```python
from build123d import *

# Parameters (mm, degrees)
SKETCH2_W           = 325
SKETCH2_H           = 220
SKETCH2_R           = 7
SKETCH2_R_2         = 3
BOSS_EXTRUDE3_DEPTH = 15
SKETCH11_W          = 70
SKETCH11_H          = 90
SKETCH11_W_2        = 50
SKETCH11_H_2        = 75
CUT_EXTRUDE2_DEPTH  = 8
FILLET1_R           = 3
SKETCH4_R           = 5
CUT_EXTRUDE3_DEPTH  = 5
SKETCH12_R          = 3
CUT_EXTRUDE4_DEPTH  = 5


with BuildPart() as part:
    # Sketch2 → Boss-Extrude3 (new body)
    with BuildSketch(Plane(origin=(0, 0, 0), x_dir=(1, 0, 0), z_dir=(0, 1, 0))):
        with Locations((7.596919738, 0)):
            Rectangle(SKETCH2_W, SKETCH2_H)
        with Locations(Location((155.096919738, -95, 0), (0, 0, 270))):
            Circle(SKETCH2_R, mode=Mode.SUBTRACT)
        with Locations(Location((155.096919738, 95, 0), (0, 0, 270))):
            Circle(SKETCH2_R, mode=Mode.SUBTRACT)
        with Locations(Location((-104.903080262, -95, 0), (0, 0, 270))):
            Circle(SKETCH2_R, mode=Mode.SUBTRACT)
        with Locations(Location((-104.903080262, 95, 0), (0, 0, 90))):
            Circle(SKETCH2_R, mode=Mode.SUBTRACT)
        with Locations(Location((-24.903080262, 105, 0), (0, 0, 270))):
            Circle(SKETCH2_R_2, mode=Mode.SUBTRACT)
        with Locations(Location((75.096919738, 105, 0), (0, 0, 270))):
            Circle(SKETCH2_R_2, mode=Mode.SUBTRACT)
        with Locations(Location((75.096919738, -105, 0), (0, 0, 90))):
            Circle(SKETCH2_R_2, mode=Mode.SUBTRACT)
        with Locations(Location((-24.903080262, -105, 0), (0, 0, 90))):
            Circle(SKETCH2_R_2, mode=Mode.SUBTRACT)
        with Locations(Location((165.096919738, 35, 0), (0, 0, 270))):
            Circle(SKETCH2_R_2, mode=Mode.SUBTRACT)
        with Locations(Location((165.096919738, -35, 0), (0, 0, 90))):
            Circle(SKETCH2_R_2, mode=Mode.SUBTRACT)
    extrude(amount=-BOSS_EXTRUDE3_DEPTH)

    # Sketch11 → Cut-Extrude2 (cut)
    with BuildSketch(Plane.XZ.offset(15)):
        with Locations((-39.903080262, 50)):
            Rectangle(SKETCH11_W, SKETCH11_H)
        with Locations((40.096919738, 50)):
            Rectangle(SKETCH11_W, SKETCH11_H)
        Polygon((85.096919738, 95), (135.096919738, 95), (135.096919738, 80), (155.096919738, 80), (155.096919738, 5), (85.096919738, 5), align=None)
        Polygon((85.096919738, -95), (85.096919738, -5), (155.096919738, -5), (155.096919738, -80), (135.096919738, -80), (135.096919738, -95), align=None)
        with Locations((40.096919738, -50)):
            Rectangle(SKETCH11_W, SKETCH11_H)
        with Locations((-39.903080262, -50)):
            Rectangle(SKETCH11_W, SKETCH11_H)
        with Locations((-109.903080262, -42.5)):
            Rectangle(SKETCH11_W_2, SKETCH11_H_2)
        with Locations((-109.903080262, 42.5)):
            Rectangle(SKETCH11_W_2, SKETCH11_H_2)
    extrude(amount=-CUT_EXTRUDE2_DEPTH, mode=Mode.SUBTRACT)

    # Fillet1
    fillet1_edges = [part.edges().sort_by_distance(p)[0] for p in [
        (85.096919738, -11, 95),
        (135.096919738, -11, 95),
        (135.096919738, -11, 80),
        (155.096919738, -11, 80),
        (155.096919738, -11, 5),
        (85.096919738, -11, 5),
        (75.096919738, -11, 5),
        (5.096919738, -11, 5),
        (5.096919738, -11, 95),
        (75.096919738, -11, 95),
        (-4.903080262, -11, 5),
        (-74.903080262, -11, 5),
        (-74.903080262, -11, 95),
        (-4.903080262, -11, 95),
        (-84.903080262, -11, 5),
        (-134.903080262, -11, 5),
        (-134.903080262, -11, 80),
        (-84.903080262, -11, 80),
        (-84.903080262, -11, -80),
        (-134.903080262, -11, -80),
        (-134.903080262, -11, -5),
        (-84.903080262, -11, -5),
        (-4.903080262, -11, -95),
        (-74.903080262, -11, -95),
        (-74.903080262, -11, -5),
        (75.096919738, -11, -95),
        (5.096919738, -11, -95),
        (5.096919738, -11, -5),
        (75.096919738, -11, -5),
        (85.096919738, -11, -95),
        (85.096919738, -11, -5),
        (155.096919738, -11, -5),
        (155.096919738, -11, -80),
        (135.096919738, -11, -80),
        (135.096919738, -11, -95),
    ]]
    fillet(fillet1_edges, radius=FILLET1_R)

    # Sketch4 → Cut-Extrude3 (cut)
    with BuildSketch(Plane(origin=(0, 0, 0), x_dir=(1, 0, 0), z_dir=(0, 1, 0))):
        with Locations(Location((-73.96287117, -44.592908869, 0), (0, 0, 270))):
            Circle(SKETCH4_R)
        with Locations(Location((81.03712883, -44.592908869, 0), (0, 0, 270))):
            Circle(SKETCH4_R)
        with Locations(Location((81.03712883, 60.407091131, 0), (0, 0, 270))):
            Circle(SKETCH4_R)
        with Locations(Location((-73.96287117, 60.407091131, 0), (0, 0, 270))):
            Circle(SKETCH4_R)
    extrude(amount=-CUT_EXTRUDE3_DEPTH, mode=Mode.SUBTRACT)

    # Sketch12 → Cut-Extrude4 (cut)
    with BuildSketch(Plane.ZY.offset(154.903080262)):
        with Locations((-102.5, -7.5)):
            Circle(SKETCH12_R)
        with Locations((-34.33, -7.5)):
            Circle(SKETCH12_R)
        with Locations((33.84, -7.5)):
            Circle(SKETCH12_R)
        with Locations((102.01, -7.5)):
            Circle(SKETCH12_R)
    extrude(amount=-CUT_EXTRUDE4_DEPTH, mode=Mode.SUBTRACT)


solid = part.part
```
Geometry check sheet. Reference: the model listing, model coordinates, mm. A direction names the side the tool comes from. Give positions to 0.01 mm unless a question says otherwise; leave off trailing zeros. Write each loop counter-clockwise with the first axis right and the second up, starting at its lowest first coordinate (ties: lowest second). Pieces come first, ordered by that corner, then holes. Notation, with made-up numbers: (14.25, 70.25) -> (28.25, 70.25) arc R31 ccw to (28.25, 105.25) -> close; hole circle Ø8 at (78, 85). An arc over 180 degrees is marked (long way). Use one line per item in the form item = value.
Item 1: Access from +Z, -Z, +X, -X, +Y, -Y to the whole of each face (thin tool, end or side, straight path). Record for faces 4 (the cylindrical face through (84.42, -2.46, -64.09)), 5 (the cylindrical face through (-152.4, -7.4, -105.5)), 6 (the flat face through (5.097, -11, -51)).
Results list:
face_4 = +Y
face_5 = -X
face_6 = -Y
Item 2: Depth check by flat-ended pin: pin 1 Ø5 at (x, z) = (165.1, -35) entering from -Y; pin 2 Ø3 at (y, z) = (-6.5, 103) entering from -X; pin 3 Ø3 at (x, z) = (-73.5, -58) entering from +Y; pin 4 Ø12 at (x, z) = (-58, -37.5) entering from -Y. Enter the tip coordinate at first touch or a pass-through.
Results list:
pin_1 = through
pin_2 = -149.9
pin_3 = -5
pin_4 = -7
Item 3: Mould release check, pull along Z, two halves, no side actions. Record for faces 1 (the flat face through (5, -7, -110)), 2 (the flat face through (5, -15, -2)), 3 (the flat face through (-134.903, -11, 42)): released by +Z, released by -Z, zero draft, split by the parting line, or undercut.
Results list:
face_1 = released by -Z
face_2 = zero draft
face_3 = undercut
Item 4: Sectioned sample at A-A on z = 15. Enter the section's corners in (x, y).
Results list:
outline = (-154.9, -15) -> (-134.9, -15) -> (-134.9, -7) -> (-84.9, -7) -> (-84.9, -15) -> (-74.9, -15) -> (-74.9, -7) -> (-4.9, -7) -> (-4.9, -15) -> (5.1, -15) -> (5.1, -7) -> (75.1, -7) -> (75.1, -15) -> (85.1, -15) -> (85.1, -7) -> (155.1, -7) -> (155.1, -15) -> (170.1, -15) -> (170.1, 0) -> (-154.9, 0) -> close
Item 5: Scan lines: line 1 (X direction, y = -10, z = -105); line 2 (X direction, y = -12.25, z = 47); line 3 (X direction, y = -6, z = -95). Record each from-to range of solid material in increasing order.
Results list:
line_1 = -154.9 to -27.9, -21.9 to 72.1, 78.1 to 170.1
line_2 = -154.9 to -134.9, -84.9 to -74.9, -4.9 to 5.1, 75.1 to 85.1, 155.1 to 170.1
line_3 = -154.9 to -111.9, -97.9 to 148.1, 162.1 to 170.1
